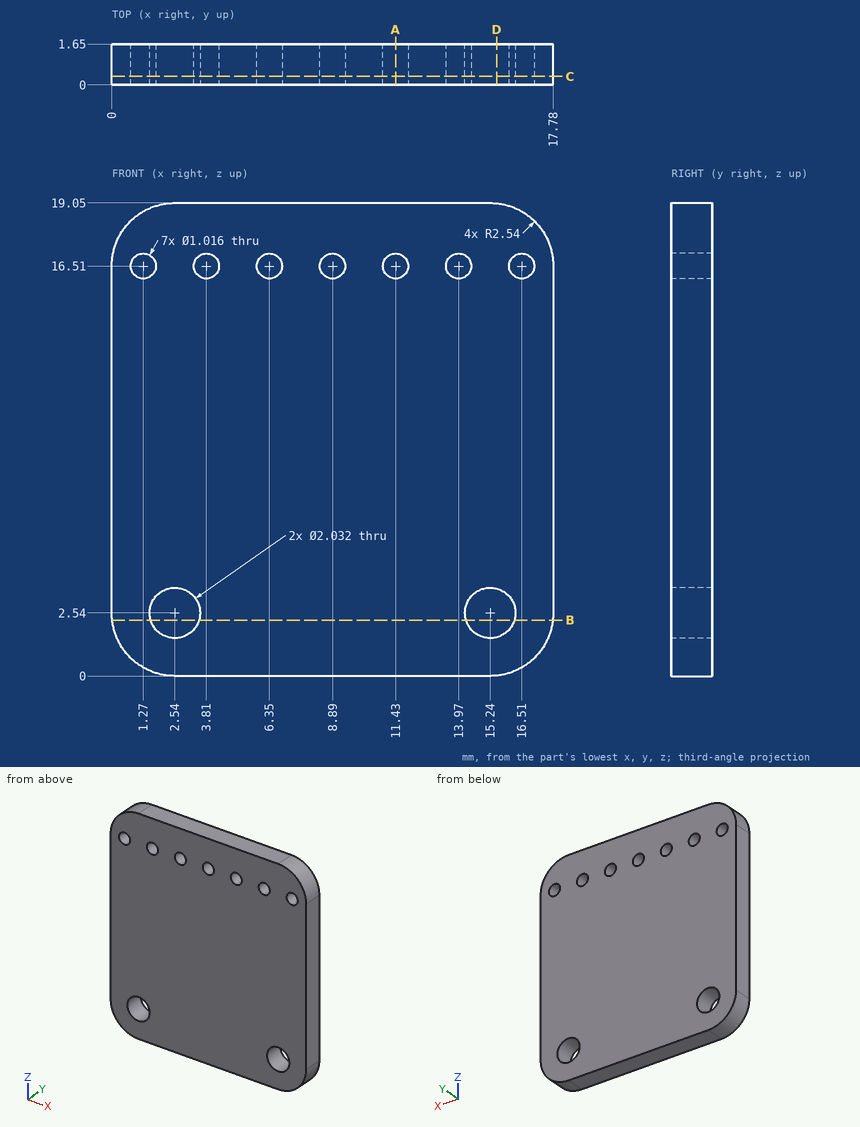
Verification items for this drawing (mm, ordinates from the low corner). Round coordinates to 2 decimals unless told otherwise and drop trailing zeros. Order: outer loops, then holes, each group sorted by start corner. A loop starts at its lowest first (then second) coordinate and runs counter-clockwise, first axis right, second up. Notation, with made-up numbers: (45, -26.75) -> (103, -26.75) arc R13 ccw to (103, -15.75) -> close; hole circle Ø7 at (44, 64.5). An arc over 180 degrees is marked (long way). Use one line per item in the form item = value.
1. Cross-section at C-C, the plane y = 0.35. Count the separate pieces of the cut face and the enclosed holes in it, plus the area to 3 significant figures.
Working result:
separate_pieces = 1
enclosed_holes = 9
area = 321 mm^2
2. Cross-section at B-B, the plane z = 2.25. Enter the section's corners in (x, y), plus the area to 3 significant figures.
Working result:
outline = (0.02, 0) -> (1.57, 0) -> (1.57, 1.65) -> (0.02, 1.65) -> close; (3.51, 0) -> (14.27, 0) -> (14.27, 1.65) -> (3.51, 1.65) -> close; (16.21, 0) -> (17.76, 0) -> (17.76, 1.65) -> (16.21, 1.65) -> close
area = 22.9 mm^2
3. Cross-section at D-D, the plane x = 15.5. Enter the section's corners in (y, z).
Working result:
outline = (0, 0.01) -> (1.65, 0.01) -> (1.65, 1.56) -> (0, 1.56) -> close; (0, 3.52) -> (1.65, 3.52) -> (1.65, 19.04) -> (0, 19.04) -> close
4. Scan lines: line 1 along X through (y, z) = (0.8, 2); line 2 along Z through (x, y) = (11.43, 1.25); line 3 along Z through (x, y) = (15.24, 0.9). Record each from-to range of solid material in increasing order. Write a range as from..to.
Working result:
line_1 = 0.06..1.68, 3.4..14.38, 16.1..17.72
line_2 = 0..16, 17.02..19.05
line_3 = 0..1.52, 3.56..19.05
5. Cross-section at A-A, the plane x = 11.43. Enter the section's corners in (y, z).
Working result:
outline = (0, 0) -> (1.65, 0) -> (1.65, 16) -> (0, 16) -> close; (0, 17.02) -> (1.65, 17.02) -> (1.65, 19.05) -> (0, 19.05) -> close
